The figure shows three views and two pictorial views of one solid part (mm, origin at its lowest corner). Answer the questions. A direction names the side the tool comes from. Coordinates: 2 decimals unless noted, no trailing zeros. Write each loop counter-clockwise with the first axis right and the second up, starting at its lowest first coordinate (ties: lowest second). Pieces come first, ordered by that corner, then holes. Notation, with made-up numbers: (59, 62) -> (103, 62) arc R29 cw to (103, 86) -> close; hole circle Ø10 at (82.5, 70.25). An arc over 180 degrees is marked (long way). Use CSV: the item, a comma, the result in double quotes. Start each with the question number.
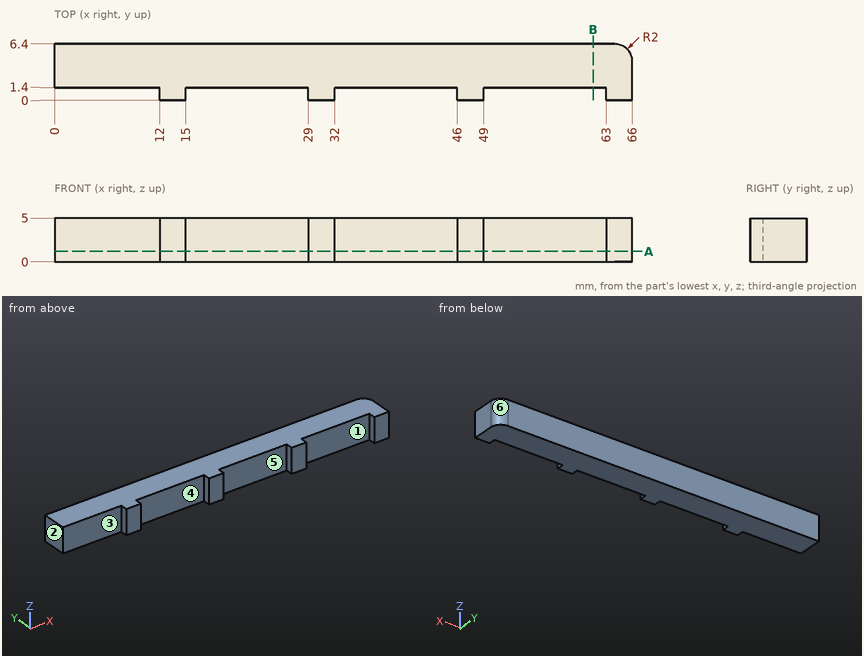
1) The mould has two halves that part along X. Classify the marked faces 1, 2, 3 and 4: pulls with the +X half, pulls with the -X half, needs draft (parallel to the pull), parting line crosses it, or undercut.
2) Find the intervals of material crossed by line 1 along X through (y, z) = (1, 0.6); line 2 along Y through (x, z) = (10, 0.75); line 3 along X through (y, z) = (4.5, 2.35), in increasing order.
3) Which of the six approach directions +Z, -Z, +X, -X, +Y, -Y give full straight-line access (tool end or side, diameter ignored) to the marked faces 5 and 6?
4) Section B-B, the plane x = 61.5 is taken. Give the vertices of the cut face in (y, z).
5) Each of these flat-tipped pins is pushed along its axis until it touches: pin 1 (1.1 mm diameter, centred on y = 1, z = 2.5, fed in from -X); pin 2 (1.5 mm diameter, centred on x = 57, z = 2.5, fed in from -Y); pin 3 (1.5 mm diameter, centred on y = 0.5, z = 2.5, fed in from -X). Where does it stop, or does it pass through?
6) Section A-A, the plane z = 1.2 is taken. Give the vertices of the cut face in (x, y).
The answers:
1,face 1,"undercut"
1,face 2,"pulls with the -X half"
1,face 3,"needs draft"
1,face 4,"undercut"
2,line 1,"x = 12 to 15, 29 to 32, 46 to 49, 63 to 66"
2,line 2,"y = 1.4 to 6.4"
2,line 3,"x = 0 to 66"
3,face 5,"+Z, -Z, -Y"
3,face 6,"+Z, -Z, +X, +Y"
4,outline,"(1.4, 0) -> (6.4, 0) -> (6.4, 5) -> (1.4, 5) -> close"
5,pin 1,"stops at x = 0"
5,pin 2,"stops at y = 1.4"
5,pin 3,"stops at x = 12"
6,outline,"(0, 1.4) -> (12, 1.4) -> (12, 0) -> (15, 0) -> (15, 1.4) -> (29, 1.4) -> (29, 0) -> (32, 0) -> (32, 1.4) -> (46, 1.4) -> (46, 0) -> (49, 0) -> (49, 1.4) -> (63, 1.4) -> (63, 0) -> (66, 0) -> (66, 4.4) arc R2 ccw to (64, 6.4) -> (0, 6.4) -> close"
